Work out the finished part from the listing and answer in its coordinate system (mm). A direction names the side the tool comes from. Coordinates: 2 decimals unless noted, no trailing zeros. Write each loop counter-clockwise with the first axis right and the second up, starting at its lowest first coordinate (ties: lowest second). Pieces come first, ordered by that corner, then holes. Notation, with made-up numbers: (-28, -9.5) - (-24, -9.5) arc R21 cw to (-24, 8.5) - close; hole circle Ø9 at (2.25, 21). An arc over 180 degrees is marked (long way). Use CSV: the item, a comma, the result in double quotes. Start each with the question number.
from build123d import *

# Parameters (mm, degrees)
BOSS_EXTRUDE1_DEPTH = 35
SKETCH2_W           = 217.526852971
SKETCH2_H           = 70
CUT_EXTRUDE1_DEPTH  = 70
CUT_EXTRUDE2_REACH  = 111.53
SKETCH3_R           = 1.5


with BuildPart() as part:
    # Sketch1 → Boss-Extrude1 (new, symmetric)
    with BuildSketch(Plane.XY):
        Polygon((0, 0), (0, 27.78), (317.526852971, 0), align=None)
    extrude(amount=BOSS_EXTRUDE1_DEPTH, both=True)

    # Sketch2 → Cut-Extrude1 (cut)
    with BuildSketch(Plane.XZ):
        with Locations((208.763426486, 0)):
            Rectangle(SKETCH2_W, SKETCH2_H)
    extrude(amount=-CUT_EXTRUDE1_DEPTH, mode=Mode.SUBTRACT)

    # Cut-Extrude2: up to this plane
    cut_extrude2_end = Plane(origin=(-0.261467228, 24.791415906, 35), z_dir=(-0.08715574274765117, -0.9961946980917462, 0))
    # Sketch3 → Cut-Extrude2 (cut, up to the surface)
    with BuildSketch(Plane.XZ, mode=Mode.PRIVATE) as cut_extrude2_sk1:
        with Locations((7, 28)):
            Circle(SKETCH3_R)
    cut_extrude2_tool1 = split(extrude(cut_extrude2_sk1.sketch, amount=-CUT_EXTRUDE2_REACH, mode=Mode.PRIVATE), bisect_by=cut_extrude2_end, keep=Keep.BOTH, mode=Mode.PRIVATE)
    add(cut_extrude2_tool1.solids().sort_by_distance((7, 0, 28))[0], mode=Mode.SUBTRACT)
    # Sketch3 → Cut-Extrude2 (cut, up to the surface)
    with BuildSketch(Plane.XZ, mode=Mode.PRIVATE) as cut_extrude2_sk2:
        with Locations((93, 28)):
            Circle(SKETCH3_R)
    cut_extrude2_tool2 = split(extrude(cut_extrude2_sk2.sketch, amount=-CUT_EXTRUDE2_REACH, mode=Mode.PRIVATE), bisect_by=cut_extrude2_end, keep=Keep.BOTH, mode=Mode.PRIVATE)
    add(cut_extrude2_tool2.solids().sort_by_distance((93, 0, 28))[0], mode=Mode.SUBTRACT)
    # Sketch3 → Cut-Extrude2 (cut, up to the surface)
    with BuildSketch(Plane.XZ, mode=Mode.PRIVATE) as cut_extrude2_sk3:
        with Locations((7, -28)):
            Circle(SKETCH3_R)
    cut_extrude2_tool3 = split(extrude(cut_extrude2_sk3.sketch, amount=-CUT_EXTRUDE2_REACH, mode=Mode.PRIVATE), bisect_by=cut_extrude2_end, keep=Keep.BOTH, mode=Mode.PRIVATE)
    add(cut_extrude2_tool3.solids().sort_by_distance((7, 0, -28))[0], mode=Mode.SUBTRACT)
    # Sketch3 → Cut-Extrude2 (cut, up to the surface)
    with BuildSketch(Plane.XZ, mode=Mode.PRIVATE) as cut_extrude2_sk4:
        with Locations((93, -28)):
            Circle(SKETCH3_R)
    cut_extrude2_tool4 = split(extrude(cut_extrude2_sk4.sketch, amount=-CUT_EXTRUDE2_REACH, mode=Mode.PRIVATE), bisect_by=cut_extrude2_end, keep=Keep.BOTH, mode=Mode.PRIVATE)
    add(cut_extrude2_tool4.solids().sort_by_distance((93, 0, -28))[0], mode=Mode.SUBTRACT)


solid = part.part
Item 1: Each of these flat-tipped pins is pushed along its axis until it touches: pin 1 (2 mm diameter, centred on x = 63.5, z = 11, fed in from +Y); pin 2 (1.8 mm diameter, centred on x = 7, z = -28, fed in from +Y); pin 3 (4 mm diameter, centred on x = 12, z = 23.5, fed in from +Y). Where does it stop, or does it pass through?
Item 2: A cutting plane is placed at C-C (y = 26.25). Determine the outline of the cut face in (x, z), then the cut area to 3 significant figures.
Item 3: Straight lines are drawn through the part: probe 1 along Z at (x, y) = (93, 9.75); probe 2 along X at (y, z) = (3.75, -28); probe 3 along X at (y, z) = (13.25, -27). For each, find the intervals that lie inside material, in ascending order. Write a range as [from, to].
Item 4: A cutting plane is placed at A-A (z = -28). Determine the outline of the cut face in (x, y).
Item 5: Which of the six approach directions +Z, -Z, +X, -X, +Y, -Y give full straight-line access (tool end or side, diameter ignored) to faces 4 (the face through (51, 11, 35)), 5 (the face through (6.805, 11.98, -26.513))?
Item 6: A cutting plane is placed at D-D (z = 14). Determine the outline of the cut face in (x, y).
Item 7: A cutting plane is placed at B-B (x = 7). Determine the outline of the cut face in (y, z).
Item 8: Determine the mould class of faces 1 (the face through (51, 11, -35)), 2 (the face through (93.806, 8.27, -26.735)), 3 (the face through (100, 9, 0)) for opening direction Z: +Z half, -Z half, draft (parallel to the pull), parting line (faces both ways), or undercut.
Calculated:
1,pin 1,"stops at y = 22.31"
1,pin 2,"stops at y = 27.25"
1,pin 3,"stops at y = 26.91"
2,outline,"(0, -35) - (17.49, -35) - (17.49, 35) - (0, 35) - close"
2,area,"1,220 mm²"
3,probe 1,"z = [-35, -29.5], [-26.5, 26.5], [29.5, 35]"
3,probe 2,"x = [0, 5.5], [8.5, 91.5], [94.5, 100]"
3,probe 3,"x = [0, 5.88], [8.12, 91.88], [94.12, 100]"
4,outline,"(0, 0) - (5.5, 0) - (5.5, 24.29) - (8.5, 24.02) - (8.5, 0) - (91.5, 0) - (91.5, 16.76) - (94.5, 16.5) - (94.5, 0) - (100, 0) - (100, 19.03) - (0, 27.78) - close"
5,face 4,"+Z, +X, -X, +Y, -Y"
5,face 5,"-Y"
6,outline,"(0, 0) - (100, 0) - (100, 19.03) - (0, 27.78) - close"
7,outline,"(0, -35) - (27.17, -35) - (27.17, 35) - (0, 35) - (0, 29.5) - (24.16, 29.5) - (24.16, 26.5) - (0, 26.5) - (0, -26.5) - (24.16, -26.5) - (24.16, -29.5) - (0, -29.5) - close"
8,face 1,"-Z half"
8,face 2,"undercut"
8,face 3,"draft"
